```python
from build123d import *

# Parameters (mm, degrees)
BOSS_EXTRUDE1_DEPTH = 10
SKETCH2_R           = 24
BOSS_EXTRUDE2_DEPTH = 12.5
SKETCH3_R           = 20
CUT_EXTRUDE1_DEPTH  = 7
CUT_EXTRUDE2_REACH  = 43.214
SKETCH4_R           = 15.5
CHAMFER1_SIZE       = 1
CHAMFER2_SIZE       = 1
CHAMFER2_SIZE2      = 0.267949192
SKETCH5_W           = 1
SKETCH5_H           = 3
FILLET1_R           = 1


with BuildPart() as part:
    # Sketch1 → Boss-Extrude1 (new body)
    with BuildSketch(Plane.XY):
        Polygon((28.867513459, 0), (14.43375673, 25), (-14.43375673, 25), (-28.867513459, 0), (-14.43375673, -25), (14.43375673, -25), align=None)
    extrude(amount=BOSS_EXTRUDE1_DEPTH)

    # Sketch2 → Boss-Extrude2 (add)
    with BuildSketch(Plane.XY.offset(10)):
        Circle(SKETCH2_R)
    extrude(amount=BOSS_EXTRUDE2_DEPTH)

    # Sketch3 → Cut-Extrude1 (cut)
    with BuildSketch(Plane(origin=(0, 0, 0), x_dir=(-1, 0, 0), z_dir=(0, 0, -1))):
        Circle(SKETCH3_R)
    extrude(amount=-CUT_EXTRUDE1_DEPTH, mode=Mode.SUBTRACT)

    # Sketch4 → Cut-Extrude2 (cut, up to next)
    with BuildSketch(Plane(origin=(0, 0, 7), x_dir=(-1, 0, 0), z_dir=(0, 0, -1)), mode=Mode.PRIVATE) as cut_extrude2_sk1:
        Circle(SKETCH4_R)
    cut_extrude2_tool1 = extrude(cut_extrude2_sk1.sketch, amount=-CUT_EXTRUDE2_REACH, mode=Mode.PRIVATE) & part.part
    add(cut_extrude2_tool1.solids().sort_by_distance((0, 0, 7))[0], mode=Mode.SUBTRACT)

    # Chamfer1
    chamfer1_edges = [part.edges().sort_by_distance(p)[0] for p in [
        (-24, 0, 22.5),
        (15.5, 0, 22.5),
        (15.5, 0, 7),
    ]]
    chamfer(chamfer1_edges, length=CHAMFER1_SIZE)

    # Chamfer2
    chamfer2_edges = [part.edges().sort_by_distance(p)[0] for p in [
        (20, 0, 0),
    ]]
    chamfer2_side = [part.faces().sort_by_distance(p)[0] for p in [
        (20, 0, 3.5),
    ]]
    chamfer(chamfer2_edges, length=CHAMFER2_SIZE, length2=CHAMFER2_SIZE2, reference=chamfer2_side[0])

    # Sketch5 → Cut-Revolve1 (revolve, cut)
    with BuildSketch(Plane(origin=(0, 0, 0), x_dir=(1, 0, 0), z_dir=(0, 1, 0))):
        Polygon((25, -10), (28.867513459, -8.963702892), (28.867513459, -10), align=None)
        with Locations((23.5, -11.5)):
            Rectangle(SKETCH5_W, SKETCH5_H)
        Polygon((28.867513459, 0), (28.867513459, -1.036297108), (25, 0), align=None)
    revolve(axis=Axis((0, 0, -102.328960849), (0, 0, 1)), mode=Mode.SUBTRACT)

    # Fillet1
    fillet1_edges = [part.edges().sort_by_distance(p)[0] for p in [
        (-23, 0, 13),
        (-23, 0, 10),
    ]]
    fillet(fillet1_edges, radius=FILLET1_R - 0.0001)  # a hair under: the kernel refuses the full size


solid = part.part
```
Part model, mm, in its own coordinate system. A direction names the side the tool comes from. Round coordinates to 2 decimals unless told otherwise and drop trailing zeros. Order: outer loops, then holes, each group sorted by start corner. A loop starts at its lowest first (then second) coordinate and runs counter-clockwise, first axis right, second up. Notation, with made-up numbers: M 83.25,-22.75 L 106.25,-22.75 A23 cw 106.25,-6.75 Z; hole C 81.5,-10.75 d8. An arc over 180 degrees is marked long. Answer in a Markdown table with one row per item. Add a question column.
Q1. Cut at B-B on z = 14. Give the cut face in (x, y).
Q2. Cut at A-A on z = 5.5. Give the cut face in (x, y).
Q3. Wall check: L1, parallel to Y at x = 0, z = 17.75; L2, parallel to X at y = -11.5, z = 10.25; L3, parallel to X at y = 6, z = 20.5. Give the ranges that are in metal, low to high. Write a range as from..to.
Q4. Mould opens along X. For faces 1 (the face through (-2.9, 16.4, 7)), 2 (the face through (-9.4, 22.3, 10)), 3 (the face through (-12.915, 22.496, 9.748)), 4 (the face through (21.75, 12.33, 4.93)) say: +X half, -X half, draft (parallel to the pull), parting line (faces both ways), or undercut.
Q5. 3-axis set-ups, long thin cutter, end or side, ignore diameter. For faces 5 (the face through (-21.55, 12.675, 4.93)), 6 (the face through (4.336, -19.524, 3.958)): which of +Z, -Z, +X, -X, +Y, -Y reach the whole face in a straight line?
Q6. Pin check, flat tips, straight feed: pin 1 (8 mm diameter, centred on y = 3.5, z = 17, fed in from -X); pin 2 (1.5 mm diameter, centred on y = -13, z = 9.5, fed in from -X) (3 decimals); pin 3 (5 mm diameter, centred on x = -21.5, z = 6, fed in from -Y); pin 4 (10 mm diameter, centred on y = 4.5, z = 5, fed in from +X). Stop position of each tip, or through.
Established:
| question | item | result |
|---|---|---|
| 1 | outline | C 0,0 d48; hole C 0,0 d31 |
| 2 | outline | M -28.87,0 L -14.43,-25 L 14.43,-25 L 28.87,0 L 14.43,25 L -14.43,25 Z; hole C 0,0 d40 |
| 3 | L1 | y = -24..-15.5, 15.5..24 |
| 3 | L2 | x = -20.31..-10.39, 10.39..20.31 |
| 3 | L3 | x = -23.24..-14.29, 14.29..23.24 |
| 4 | face 1 | undercut |
| 4 | face 2 | draft |
| 4 | face 3 | -X half |
| 4 | face 4 | +X half |
| 5 | face 5 | +Z, -Z, -X, +Y |
| 5 | face 6 | -Z |
| 6 | pin 1 | stops at x = -24 |
| 6 | pin 2 | stops at x = -21.795 |
| 6 | pin 3 | stops at y = -17.09 |
| 6 | pin 4 | stops at x = 28.87 |
